Check sheet for the modelled part. Datum: model origin and axes. Units: mm. A direction names the side the tool comes from. Give positions to 0.01 mm unless a question says otherwise; leave off trailing zeros. Order: outer loops, then holes, each group sorted by start corner. A loop starts at its lowest first (then second) coordinate and runs counter-clockwise, first axis right, second up. Notation, with made-up numbers: (14, 18.25) -> (26, 18.25) arc R8 cw to (26, 29.25) -> close; hole circle Ø1 at (4, -38.5). An arc over 180 degrees is marked (long way). Answer in a Markdown table with one row per item. Add a question column.
(1) Release check for a two-part mould opening along X. For faces 1 (the face through (3.9, 1.5, -0.3)), 2 (the face through (6.51, -1.48, -7.51)), 3 (the face through (4, 0.4, -4)) record: released by +X, released by -X, zero draft, split by the parting line, or undercut.
(2) Cross-section at B-B (x = 4). Record the cut outline in (y, z).
(3) Cross-section at C-C (y = 0.9). Record the cut outline in (x, z), then the cut area to 3 significant figures.
(4) Set-up check for faces 4 (the face through (2.94, 0.2, -2.36)), 5 (the face through (1.49, -1.48, -7.49)), 6 (the face through (4.409, 2.803, -4.075)), 7 (the face through (3, 0, -2)): record each of +Z, -Z, +X, -X, +Y, -Y from which the full face is reachable in a straight line by a thin tool's end or side.
(5) Thickness scan on L1, parallel to Y at x = 6.75, z = -6; L2, parallel to X at y = 0.3, z = -3.75; L3, parallel to Y at x = 3, z = -4.25. Record the ranges inside material, lowest first. Write a range as [from, to].
(6) Cross-section at A-A (z = -3.75). Record the cut outline in (x, y).
(7) Go/stop test with flat-tipped pins: pin 1 (1 mm diameter, centred on y = 1.5, z = -4.5, fed in from +X); pin 2 (2.5 mm diameter, centred on x = 4, z = -4, fed in from +Y); pin 3 (2 mm diameter, centred on x = 2, z = -2.5, fed in from -Y); pin 4 (2 mm diameter, centred on x = 2.5, y = 2.5, fed in from +Z). Record where each tip stops, or that it passes through.
(8) Cross-section at D-D (x = 1.5). Record the cut outline in (y, z).
```python
from build123d import *

# Parameters (mm, degrees)
SKETCH1_W               = 8
SKETCH1_H               = 8
BOSS_EXTRUDE1_DEPTH     = 3
CUT_EXTRUDE1_DEPTH      = 12.704699911
CUT_EXTRUDE1_DEPTH_BACK = 12.704699911
CUT_EXTRUDE2_DEPTH      = 11
SKETCH4_R               = 1.75
CUT_EXTRUDE3_DEPTH      = 0.4
SKETCH5_W               = 8
SKETCH5_H               = 1
BOSS_EXTRUDE2_DEPTH     = 2
FILLET1_R               = 4
CUT_EXTRUDE4_DEPTH      = 0.4


with BuildPart() as part:
    # Sketch1 → Boss-Extrude1 (new body)
    with BuildSketch(Plane(origin=(0, 0, 0), x_dir=(1, 0, 0), z_dir=(0, 1, 0))):
        with Locations((4, 4)):
            Rectangle(SKETCH1_W, SKETCH1_H)
    extrude(amount=BOSS_EXTRUDE1_DEPTH)

    # Sketch2 → Cut-Extrude1 (cut, two sides: drawn at the far end of the back side and taken through both)
    with BuildSketch(Plane.XY.offset(-CUT_EXTRUDE1_DEPTH_BACK)):
        Polygon((0, 0), (0.6, 3), (0, 3), align=None)
        Polygon((8, 0), (7.4, 3), (8, 3), align=None)
    extrude(amount=CUT_EXTRUDE1_DEPTH + CUT_EXTRUDE1_DEPTH_BACK, mode=Mode.SUBTRACT)

    # Sketch3 → Cut-Extrude2 (cut)
    with BuildSketch(Plane(origin=(0, 0, 0), x_dir=(0, 0, -1), z_dir=(1, 0, 0))):
        Polygon((0, 0), (0.6, 3), (0, 3), align=None)
        Polygon((8, 3), (7.4, 3), (8, 0), align=None)
    extrude(amount=CUT_EXTRUDE2_DEPTH, mode=Mode.SUBTRACT)

    # Sketch4 → Cut-Extrude3 (cut)
    with BuildSketch(Plane.XZ):
        with Locations(Location((4, -3.75, 0), (0, 0, 270))):
            Circle(SKETCH4_R)
    extrude(amount=-CUT_EXTRUDE3_DEPTH, mode=Mode.SUBTRACT)

    # Sketch5 → Boss-Extrude2 (add)
    with BuildSketch(Plane.XZ):
        with Locations((4, -7.5)):
            Rectangle(SKETCH5_W, SKETCH5_H)
    extrude(amount=BOSS_EXTRUDE2_DEPTH)

    # Fillet1
    # the kernel refuses this fillet: 4 mm, written as the material it takes off along each edge
    with BuildSketch(Plane(origin=(8, -2, -16.660254038), x_dir=(0, 1, 0), z_dir=(0, 0, 1)), Plane(origin=(0, -2, 1.660254038), x_dir=(0, 1, 0), z_dir=(0, 0, -1))) as fillet1_piece_1:
        with BuildLine():
            CenterArc((4, 3.464101615), FILLET1_R, 180, 60)
            Line((0, 3.464101615), (-0.08, 3.464101615))
            Line((-0.08, 3.464101615), (-0.08, 0))
            Line((-0.08, 0), (0, -0.08))
            ThreePointArc((0, -0.08), (1, -0.08), (1.96, -0.069282032))
            Line((1.96, -0.069282032), (2, 0))
        make_face()
    extrude(amount=18.320508076, mode=Mode.SUBTRACT)

    # Sketch6 → Cut-Extrude4 (cut)
    with BuildSketch(Plane(origin=(0, 3, 0), x_dir=(1, 0, 0), z_dir=(0, 1, 0))):
        Polygon((2.33946821, 2.056832464), (2.33946821, 2.774781182), (4.546198979, 5.390165797), (2.595878466, 5.390165797), (2.595878466, 6.056832464), (5.518955389, 6.056832464), (5.518955389, 5.390165797), (3.268154107, 2.72349913), (5.570237441, 2.72349913), (5.570237441, 2.056832464), align=None)
    extrude(amount=-CUT_EXTRUDE4_DEPTH, mode=Mode.SUBTRACT)


solid = part.part
```
Answer below:
| question | item | result |
|---|---|---|
| 1 | face 1 | zero draft |
| 1 | face 2 | released by +X |
| 1 | face 3 | undercut |
| 2 | outline | (-2, -8) -> (0, -8) -> (3, -7.4) -> (3, -6.06) -> (2.6, -6.06) -> (2.6, -5.39) -> (3, -5.39) -> (3, -4.74) -> (2.6, -4.74) -> (2.6, -3.59) -> (3, -3.59) -> (3, -2.72) -> (2.6, -2.72) -> (2.6, -2.06) -> (3, -2.06) -> (3, -0.6) -> (0, 0) -> (0, -2) -> (0.4, -2) -> (0.4, -5.5) -> (0, -5.5) -> (0, -7) -> (-2, -7) -> close |
| 3 | outline | (0.18, -7.82) -> (7.82, -7.82) -> (7.82, -0.18) -> (0.18, -0.18) -> close |
| 3 | area | 58.4 mm² |
| 4 | face 4 | -Y |
| 4 | face 5 | +Z, -Z, -X, -Y |
| 4 | face 6 | +Y |
| 4 | face 7 | +Z, +X, -X, -Y |
| 5 | L1 | y = [0, 3] |
| 5 | L2 | x = [0.06, 2.25], [5.75, 7.94] |
| 5 | L3 | y = [0.4, 3] |
| 6 | outline | (0, 0) -> (2.25, 0) -> (2.25, 0.4) -> (5.75, 0.4) -> (5.75, 0) -> (8, 0) -> (7.4, 3) -> (4.13, 3) -> (4.13, 2.6) -> (3.16, 2.6) -> (3.16, 3) -> (0.6, 3) -> close |
| 7 | pin 1 | stops at x = 7.8 |
| 7 | pin 2 | stops at y = 3 |
| 7 | pin 3 | stops at y = 0 |
| 7 | pin 4 | stops at z = -0.3 |
| 8 | outline | (-1.48, -8) -> (0, -8) -> (3, -7.4) -> (3, -0.6) -> (0, 0) -> (0, -7) -> (-1.48, -7) -> close |
